Geometry check sheet. Reference: the model listing, model coordinates, mm. Give positions to 0.01 mm unless a question says otherwise; leave off trailing zeros. Write each loop counter-clockwise with the first axis right and the second up, starting at its lowest first coordinate (ties: lowest second). Pieces come first, ordered by that corner, then holes. Notation, with made-up numbers: (73, 5) - (81, 5) arc R31 cw to (81, 32) - close; hole circle Ø2 at (-40, 85). An arc over 180 degrees is marked (long way). Use a Markdown table: item, result.
Autodesk Inventor part; units mm, degrees
ref_plane "Work Plane1" through (0, 0, 0) normal (0, -1, 0) x (1, 0, 0)
ref_plane "YZ Plane" through (0, 0, 0) normal (1, 0, 0) x (0, 1, 0)
ref_plane "XZ Plane" through (0, 0, 0) normal (0, 1, 0) x (-1, 0, 0)
sketch "Sketch1" plane through (0, 0, 0) normal (1, 0, 0) x (0, 1, 0)
  circle A0 centre (0, 0) radius 3.35
  circle A1 centre (0, 0) radius 1.95
  dimension "d0" = 3.9
  dimension "d1" = 6.7
extrude "Body" add sketch "Sketch1" along normal blind 0.7
fillet "Fillet" radius 0.1 2 edges at (0.7, -1.95, 0) (0, -1.95, 0)
sketch "Sketch2" plane through (0, 0, 0) normal (0, 0, 1) x (1, 0, 0)
  line L0 (0, -1.95) -> (0, 1.95)
  line L1 (0.7, 3.35) -> (0.7, -3.35)
  line L2 (-1.2, 0) -> (7.2, 0)
  line L3 (0, -0.14) -> (0.7, 0.2641)
  line L4 (0, 0.14) -> (0.7, 0.5441)
  dimension "d4" = 0.14
  dimension "d5" = 0.14
  dimension "d6" = 60
extrude "Cut" cut sketch "Sketch2" along normal up to next contours L0 L2 L3 | L0 L4 L1 L3 L2
ref_plane "Work Plane1" through (0, 0, 0) normal (0, -1, 0) x (1, 0, 0)
equation "\"d0\" = SD1"
equation "\"d1\" = SD2"
equation "\"d2\" = SD"
equation "\"d4\" = 0.2 * SD"
equation "\"d5\" = 0.2 * SD"
equation "\"d6\" = FAWI"
equation "\"d7\" = SD"
equation "\"d13\" = R"
equation "\"SD1\" = 3.9"
equation "\"SD2\" = 6.7"
equation "\"SD\" = 0.7"
equation "\"FAWI\" = 60deg"
equation "\"R\" = 0.1"
equation "\"NND\" = 3.5"
properties part number "DIN 128 - A3.5" material "Steel, Mild"
1) Section check A-A on y = 0. Record the boundary of the cut face in (x, z), then the cut area to 3 significant figures.
Working result:
| item | result |
|---|---|
| outline | (0, -3.35) - (0.7, -3.35) - (0.7, -2.05) arc R0.1 ccw to (0.6, -1.95) - (0.1, -1.95) arc R0.1 ccw to (0, -2.05) - close; (0.24, 1.95) - (0.6, 1.95) arc R0.1 ccw to (0.7, 2.05) - (0.7, 3.35) - (0.24, 3.35) - close |
| area | 1.61 mm² |
2) Section check B-B on z = 2.25. Record the boundary of the cut face in (x, y), then the cut area to 3 significant figures.
Working result:
| item | result |
|---|---|
| outline | (0, -2.48) - (0.7, -2.48) - (0.7, 0.26) - (0, -0.14) - close; (0, 0.14) - (0.7, 0.54) - (0.7, 2.48) - (0, 2.48) - close |
| area | 3.28 mm² |
3) Section check D-D on y = 2.25. Record the boundary of the cut face in (x, z).
Working result:
| item | result |
|---|---|
| outline | (0, -2.48) - (0.7, -2.48) - (0.7, 2.48) - (0, 2.48) - close |
4) Section check C-C on x = 0.3. Record the boundary of the cut face in (y, z).
Working result:
| item | result |
|---|---|
| outline | (0.03, 1.95) - (0.03, 3.35) arc R3.35 ccw (long way) to (0.31, 3.34) - (0.31, 1.92) arc R1.95 cw (long way) to start |
5) Material ranges on L1, parallel to Z at x = 0.55, y = 0; L2, parallel to Y at x = 0.6, z = 1.75, recorded low to high. Write a range as from..to.
Working result:
| item | result |
|---|---|
| L1 | z = -3.35..-1.95, 1.95..3.35 |
| L2 | y = -2.86..-0.86, 0.86..2.86 |
